Input: part model. Units: mm. Frame: model coordinates. A direction names the side the tool comes from. Give positions to 0.01 mm unless a question says otherwise; leave off trailing zeros. Order: outer loops, then holes, each group sorted by start corner. A loop starts at its lowest first (then second) coordinate and runs counter-clockwise, first axis right, second up. Notation, with made-up numbers: M 5,-37 L 20,-37 A14 ccw 20,-21 Z; hole C 87,50 d3. An arc over 180 degrees is marked long. Use a Markdown table: item, result.
from build123d import *

# Parameters (mm, degrees)
SZKIC1_R                   = 9
WYCI_GNI_CIE1_DEPTH        = 12
SZKIC2_R                   = 6
WYCI_GNI_CIE2_DEPTH        = 30
WYTNIJ_WYCI_GNI_CIE1_DEPTH = 7
SZKIC4_R                   = 5.810938268
WYTNIJ_WYCI_GNI_CIE2_DEPTH = 2
WYTNIJ_WYCI_GNI_CIE2_DRAFT = -45
ZAOKR_GLENIE1_R            = 1
SFAZOWANIE1_SIZE           = 1


with BuildPart() as part:
    # Szkic1 → Wyciągnięcie1 (new body)
    with BuildSketch(Plane(origin=(0, 0, 0), x_dir=(1, 0, 0), z_dir=(0, 1, 0))):
        with Locations(Location((0, 0, 0), (0, 0, 270))):
            Circle(SZKIC1_R)
    extrude(amount=WYCI_GNI_CIE1_DEPTH)

    # Szkic2 → Wyciągnięcie2 (add)
    with BuildSketch(Plane.XZ):
        with Locations(Location((0, 0, 0), (0, 0, 90))):
            Circle(SZKIC2_R)
    extrude(amount=WYCI_GNI_CIE2_DEPTH)

    # Szkic3 → Wytnij-wyciągnięcie1 (cut)
    with BuildSketch(Plane(origin=(0, 12, 0), x_dir=(-1, 0, 0), z_dir=(0, 1, 0))):
        Polygon((0, 5.773502692), (-5, 2.886751346), (-5, -2.886751346), (0, -5.773502692), (5, -2.886751346), (5, 2.886751346), align=None)
    extrude(amount=-WYTNIJ_WYCI_GNI_CIE1_DEPTH, mode=Mode.SUBTRACT)


with BuildPart() as wytnij_wyci_gni_cie2_tool:
    # Szkic4 → Wytnij-wyciągnięcie2 (with draft: the straight prism first)
    with BuildSketch(Plane(origin=(0, 12, 0), x_dir=(-1, 0, 0), z_dir=(0, 1, 0))):
        Circle(SZKIC4_R)
    extrude(amount=-WYTNIJ_WYCI_GNI_CIE2_DEPTH)
    # Wytnij-wyciągnięcie2: the draft: its side faces are tilted about the plane it starts from
    wytnij_wyci_gni_cie2_sides = [wytnij_wyci_gni_cie2_tool.faces().sort_by_distance(p)[0] for p in [
        (5.810938268, 11, 0),
    ]]
    draft(wytnij_wyci_gni_cie2_sides, Plane(origin=(0, 12, 0), x_dir=(-1, 0, 0), z_dir=(0, 1, 0)), WYTNIJ_WYCI_GNI_CIE2_DRAFT)


with BuildPart() as part_1:
    add(part.part)

    # Wytnij-wyciągnięcie2: cut by wytnij_wyci_gni_cie2_tool
    add(wytnij_wyci_gni_cie2_tool.part, mode=Mode.SUBTRACT)

    # Zaokrąglenie1
    zaokr_glenie1_edges = [part_1.edges().sort_by_distance(p)[0] for p in [
        (0, 12, -9),
    ]]
    fillet(zaokr_glenie1_edges, radius=ZAOKR_GLENIE1_R)

    # Sfazowanie1
    sfazowanie1_edges = [part_1.edges().sort_by_distance(p)[0] for p in [
        (0, -30, -6),
    ]]
    chamfer(sfazowanie1_edges, length=SFAZOWANIE1_SIZE)


solid = part_1.part
1) Reachability of faces 4 (the face through (-2.535, 8.53, 4.31)), 5 (the face through (5, 12, 4)), 6 (the face through (-1.802, -14.297, 5.723)) from +Z, -Z, +X, -X, +Y, -Y: full face, straight path, thin tool, end or side. Return the list, or none.
Response values:
| item | result |
|---|---|
| face 4 | +Y |
| face 5 | +Z, -Z, +X, -X, +Y |
| face 6 | -Y |
2) Material intervals for line 1 (Z direction, x = 1.5, y = -5); line 2 (Y direction, x = 3, z = -3.5); line 3 (Y direction, x = -5, z = 4), sorted ascending. Write a range as from..to.
Response values:
| item | result |
|---|---|
| line 1 | z = -5.81..5.81 |
| line 2 | y = -30..5 |
| line 3 | y = 0..12 |
3) Cut plane A-A on z = 0. Return loops of the section in (x, y), and give its area (3 significant figures).
Response values:
| item | result |
|---|---|
| outline | M -9,0 L -6,0 L -6,-29 L -5,-30 L 5,-30 L 6,-29 L 6,0 L 9,0 L 9,11 A1 ccw 8,12 L 5.81,12 L 5,11.19 L 5,5 L -5,5 L -5,11.19 L -5.81,12 L -8,12 A1 ccw -9,11 Z |
| area | 504 mm² |
4) Mould query, pull axis X, two halves, no side actions, for faces 1 (the face through (2.703, 5.423, 8.584)), 2 (the face through (0, -30, 0)), 3 (the face through (2.465, 8.53, 4.35)). Classes: released by +X, released by -X, zero draft, split by the parting line, or undercut.
Response values:
| item | result |
|---|---|
| face 1 | split by the parting line |
| face 2 | zero draft |
| face 3 | undercut |
5) First-contact query: pin 1 Ø8 at (y, z) = (-1, -6) entering from +X; pin 2 Ø2 at (y, z) = (-6, 5.5) entering from -X; pin 3 Ø1 at (x, z) = (-4, 5.5) entering from -Y. Flat tips, straight axial feed; report the tip coordinate or a pass-through.
Response values:
| item | result |
|---|---|
| pin 1 | stops at x = 8.75 |
| pin 2 | stops at x = -3.97 |
| pin 3 | stops at y = 0 |
6) Cut plane B-B on y = -8. Return loops of the section in (x, z), and give its area (3 significant figures).
Response values:
| item | result |
|---|---|
| outline | C 0,0 d12 |
| area | 113 mm² |
